from build123d import *

# Parameters (mm, degrees)
SKETCH1_W               = 76.2
SKETCH1_H               = 44.45
BOSS_EXTRUDE1_DEPTH     = 9.525
F_1_CLEARANCE_HOLE1_D   = 26.19248
F_1_4_CLEARANCE_HOLE1_D = 6.7564


with BuildPart() as part:
    # Sketch1 → Boss-Extrude1 (new body)
    with BuildSketch(Plane.XY):
        Rectangle(SKETCH1_W, SKETCH1_H)
    extrude(amount=BOSS_EXTRUDE1_DEPTH)

    # 1 Clearance Hole1 (through all)
    with Locations(Plane.XY.offset(9.525)):
        with Locations((0, 0)):
            Hole(F_1_CLEARANCE_HOLE1_D / 2)

    # 1/4 Clearance Hole1 (through all)
    with Locations(Plane.XY.offset(9.525)):
        with Locations((-28.575, 0), (28.575, 0)):
            Hole(F_1_4_CLEARANCE_HOLE1_D / 2)


solid = part.part
The listing builds one solid part. Answer for the finished solid, in the listing's coordinates (mm). Coordinates: 2 decimals unless noted, no trailing zeros. Loops run counter-clockwise (first coordinate to the right, second up) from the corner with the lowest first, then second, coordinate; pieces in that order, holes last.
1) Find the intervals of material crossed by L1, parallel to Y at x = -28.5, z = 1.5 (3 decimals); L2, parallel to Y at x = -2.5, z = 0.75 (3 decimals); L3, parallel to X at y = -4, z = 5, in increasing order.
2) Find section C-C on y = 6.5. Write down the section's boundary in (x, z) (3 decimals).
3) Find section B-B on z = 2.5. Write down the section's boundary in (x, y) (3 decimals), then the cut area to 3 significant figures.
4) Find section A-A on x = 0. Write down the section's boundary in (y, z) (3 decimals).
5) Find section D-D on y = 0. Write down the section's boundary in (x, z) (3 decimals), then the cut area to 3 significant figures.
6) Determine the mould class of faces 1 (the face through (38.1, 0, 5)), 2 (the face through (-9, 10, 0)), 3 (the face through (-31.696, -1.294, 4.696)) for opening direction X: pulls with the +X half, pulls with the -X half, needs draft (parallel to the pull), parting line crosses it, or undercut.
Values:
1. L1: y = -22.225 to -3.377, 3.377 to 22.225
1. L2: y = -22.225 to -12.855, 12.855 to 22.225
1. L3: x = -38.1 to -12.47, 12.47 to 38.1
2. outline: (-38.1, 0) - (-11.369, 0) - (-11.369, 9.525) - (-38.1, 9.525) - close; (11.369, 0) - (38.1, 0) - (38.1, 9.525) - (11.369, 9.525) - close
3. outline: (-38.1, -22.225) - (38.1, -22.225) - (38.1, 22.225) - (-38.1, 22.225) - close; hole circle Ø6.756 at (-28.575, 0); hole circle Ø26.192 at (0, 0); hole circle Ø6.756 at (28.575, 0)
3. area: 2,780 mm2
4. outline: (-22.225, 0) - (-13.096, 0) - (-13.096, 9.525) - (-22.225, 9.525) - close; (13.096, 0) - (22.225, 0) - (22.225, 9.525) - (13.096, 9.525) - close
5. outline: (-38.1, 0) - (-31.953, 0) - (-31.953, 9.525) - (-38.1, 9.525) - close; (-25.197, 0) - (-13.096, 0) - (-13.096, 9.525) - (-25.197, 9.525) - close; (13.096, 0) - (25.197, 0) - (25.197, 9.525) - (13.096, 9.525) - close; (31.953, 0) - (38.1, 0) - (38.1, 9.525) - (31.953, 9.525) - close
5. area: 348 mm2
6. face 1: pulls with the +X half
6. face 2: needs draft
6. face 3: undercut
